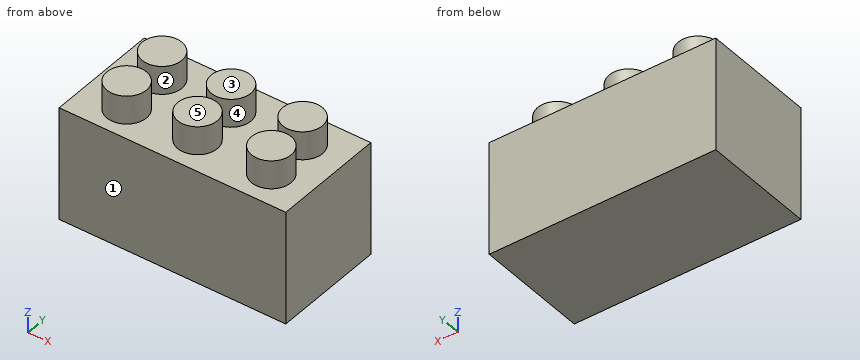
from build123d import *

# Parameters (mm, degrees)
F0_W     = 25.4
F0_H     = 12.7
F1_DEPTH = 12.7
F2_R     = 2.2225
F3_DEPTH = 3.175


with BuildPart() as f1:
    # F0 (on Front) → F1 (new body)
    with BuildSketch(Plane.XZ):
        Rectangle(F0_W, F0_H)
    extrude(amount=F1_DEPTH)

    # F2 (on face) → F3 (join)
    with BuildSketch(Plane.XY.offset(6.35)):
        with Locations((-7.762069, -9.199759)):
            Circle(F2_R)
        with Locations((0, -8.961292)):
            Circle(F2_R)
        with Locations((8.274858, -8.961292)):
            Circle(F2_R)
        with Locations((7.976773, -3.893862)):
            Circle(F2_R)
        with Locations((0, -3.953478)):
            Circle(F2_R)
        with Locations((-7.821687, -3.834245)):
            Circle(F2_R)
    extrude(amount=F3_DEPTH)


solid = f1.part
Verification items for the finished model (mm, model axes). Face numbers are marked on the shaded views. A direction names the side the tool comes from. Coordinates: 2 decimals unless noted, no trailing zeros. Write each loop counter-clockwise with the first axis right and the second up, starting at its lowest first coordinate (ties: lowest second). Pieces come first, ordered by that corner, then holes. Notation, with made-up numbers: M 26,43.5 L 48,43.5 A23 ccw 48,62.5 Z; hole C -30.5,84.5 d1. An arc over 180 degrees is marked long. One line per question, with ' | ' between items.
1) Sectioned sample at D-D on y = -4.5. Record the cut outline in (x, z) (3 decimals).
Solutions:
outline: M -12.7,-6.35 L 12.7,-6.35 L 12.7,6.35 L 10.115,6.35 L 10.115,9.525 L 5.839,9.525 L 5.839,6.35 L 2.154,6.35 L 2.154,9.525 L -2.154,9.525 L -2.154,6.35 L -5.701,6.35 L -5.701,9.525 L -9.942,9.525 L -9.942,6.35 L -12.7,6.35 Z
2) Material ranges on L1, parallel to X at y = -2, z = 6.75; L2, parallel to Z at x = 2.5, y = -1; L3, parallel to X at y = -10, z = 6.5, recorded low to high.
Solutions:
L1: -9.08 to -6.57, -1.06 to 1.06, 6.81 to 9.14 | L2: -6.35 to 6.35 | L3: -9.84 to -5.69, -1.96 to 1.96, 6.31 to 10.24
3) Sectioned sample at B-B on y = -2.5. Record the cut outline in (x, z) (3 decimals), then the cut area to 3 significant figures.
Solutions:
outline: M -12.7,-6.35 L 12.7,-6.35 L 12.7,6.35 L 9.708,6.35 L 9.708,9.525 L 6.246,9.525 L 6.246,6.35 L 1.681,6.35 L 1.681,9.525 L -1.681,9.525 L -1.681,6.35 L -6.044,6.35 L -6.044,9.525 L -9.599,9.525 L -9.599,6.35 L -12.7,6.35 Z | area: 356 mm^2
4) Access from +Z, -Z, +X, -X, +Y, -Y to the whole of each face (thin tool, end or side, straight path). Record for the marked faces 4 and 5.
Solutions:
face 4: +Z | face 5: +Z, +X, -X, +Y, -Y
5) Sectioned sample at C-C on z = 7.5. Record the cut outline in (x, y) (1 decimal), then the cut area to 3 significant figures.
Solutions:
outline: C -7.8,-9.2 d4.4; C -7.8,-3.8 d4.4; C 0,-9 d4.4; C 0,-4 d4.4; C 8,-3.9 d4.4; C 8.3,-9 d4.4 | area: 93.1 mm^2
6) Sectioned sample at A-A on x = 0. Record the cut outline in (y, z) (3 decimals), then the cut area to 3 significant figures.
Solutions:
outline: M -12.7,-6.35 L 0,-6.35 L 0,6.35 L -1.731,6.35 L -1.731,9.525 L -6.176,9.525 L -6.176,6.35 L -6.739,6.35 L -6.739,9.525 L -11.184,9.525 L -11.184,6.35 L -12.7,6.35 Z | area: 190 mm^2
7) Depth check by flat-ended pin: pin 1 Ø8 at (x, z) = (4, 1.5) entering from +Y. Enter the tip coordinate at first touch or a pass-through.
Solutions:
pin 1: y = 0
8) Release check for a two-part mould opening along Y. For the marked faces 1, 2 and 3 record: +Y half, -Y half, draft (parallel to the pull), parting line (faces both ways), or undercut.
Solutions:
face 1: -Y half | face 2: undercut | face 3: draft
